Design review of the part built by this model. Coordinates are the model's own, in mm. Coordinates: 2 decimals unless noted, no trailing zeros. Write each loop counter-clockwise with the first axis right and the second up, starting at its lowest first coordinate (ties: lowest second). Pieces come first, ordered by that corner, then holes.
Q1. Add section B-B, the plane x = 4.75. Give the boundary of the cut face in (y, z), plus the area to 3 significant figures.
Q2. To check wall thickness, follow probe 1 along Z at (x, y) = (8.5, 0); probe 2 along Y at (x, z) = (5, -28); probe 3 along Z at (x, y) = (2.25, -2.25). State the ranges of each line that lie inside material, in increasing order.
Q3. Add section C-C, the plane z = 40. Give the boundary of the cut face in (x, y), plus the area to 3 significant figures.
Q4. The part is to be moulded in two halves that separate along Y. For faces 1 (the face through (12, 0, 1)), 2 (the face through (6, 12.5, -1)), 3 (the face through (6, 0, -26)), 4 (the face through (6.084, 0.521, 36.034)), say which applies: +Y half, -Y half, draft (parallel to the pull), parting line (faces both ways), or undercut.
Q5. Add section A-A, the plane z = -28. Give the boundary of the cut face in (x, y).
from build123d import *

# Parameters (mm, degrees)
F0_W     = 25
F0_H     = 108
F1_DEPTH = 12
F2_D     = 8
F3_D     = 4


with BuildPart() as f1:
    # F0 (on Right) → F1 (new body)
    with BuildSketch(Plane.YZ):
        Rectangle(F0_W, F0_H)
    extrude(amount=F1_DEPTH)

    # F2 (through all)
    with Locations(Plane(origin=(0, 0, 0), x_dir=(0, 1, 0), z_dir=(-1, 0, 0))):
        with Locations((0, -40), (0, 40)):
            Hole(F2_D / 2)

    # F3 (through all)
    with Locations(Plane(origin=(0, 0, 0), x_dir=(0, 1, 0), z_dir=(-1, 0, 0))):
        with Locations((0, 28)):
            Hole(F3_D / 2)


solid = f1.part
Here are the results:
1. outline: (-12.5, -54) - (12.5, -54) - (12.5, 54) - (-12.5, 54) - close; hole circle Ø8 at (0, -40); hole circle Ø8 at (0, 40); hole circle Ø4 at (0, -28)
1. area: 2,590 mm2
2. probe 1: z = -54 to -44, -36 to -30, -26 to 36, 44 to 54
2. probe 2: y = -12.5 to -2, 2 to 12.5
2. probe 3: z = -54 to -43.31, -36.69 to 36.69, 43.31 to 54
3. outline: (0, -12.5) - (12, -12.5) - (12, -4) - (0, -4) - close; (0, 4) - (12, 4) - (12, 12.5) - (0, 12.5) - close
3. area: 204 mm2
4. face 1: draft
4. face 2: +Y half
4. face 3: undercut
4. face 4: undercut
5. outline: (0, -12.5) - (12, -12.5) - (12, -2) - (0, -2) - close; (0, 2) - (12, 2) - (12, 12.5) - (0, 12.5) - close
